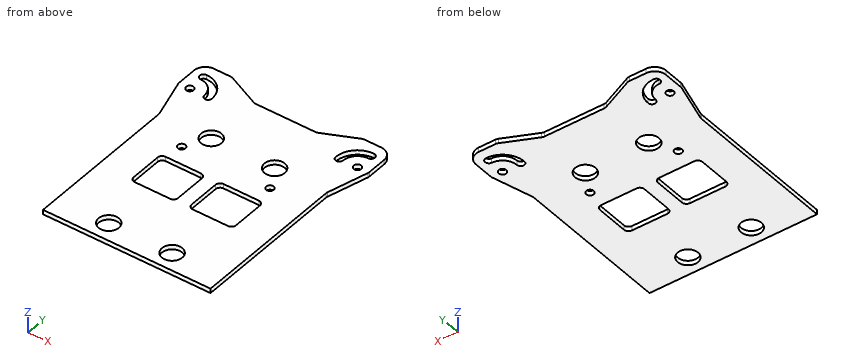
from build123d import *

# Parameters (mm, degrees)
F0_R     = 4.5
F0_R_2   = 1.65
F1_DEPTH = 2


with BuildPart() as f1:
    # F0 (on Top) → F1 (new body)
    with BuildSketch(Plane.XY):
        with BuildLine():
            Line((-29.655639, 60.219758), (-37, 60.219758))
            ThreePointArc((-37, 60.219758), (-40.535534, 58.755292), (-42, 55.219758))
            Line((-42, 55.219758), (-42, 46.628683))
            ThreePointArc((-42, 46.628683), (-41.972513, 46.223505), (-41.890554, 45.825751))
            Line((-41.890554, 45.825751), (-37.109446, 28.613764))
            ThreePointArc((-37.109446, 28.613764), (-37.027487, 28.216011), (-37, 27.810833))
            Line((-37, 27.810833), (-37, -39.780242))
            Line((-37, -39.780242), (37, -39.780242))
            Line((37, -39.780242), (37, 27.810833))
            ThreePointArc((37, 27.810833), (37.027487, 28.216011), (37.109446, 28.613764))
            Line((37.109446, 28.613764), (41.890554, 45.825751))
            ThreePointArc((41.890554, 45.825751), (41.972513, 46.223505), (42, 46.628683))
            Line((42, 46.628683), (42, 55.219758))
            ThreePointArc((42, 55.219758), (40.535534, 58.755292), (37, 60.219758))
            Line((37, 60.219758), (29.655639, 60.219758))
            ThreePointArc((29.655639, 60.219758), (29.015118, 60.150582), (28.404136, 59.946246))
            Line((28.404136, 59.946246), (14.345864, 53.493269))
            ThreePointArc((14.345864, 53.493269), (13.734882, 53.288933), (13.094361, 53.219758))
            Line((13.094361, 53.219758), (0, 53.219758))
            Line((0, 53.219758), (-13.094361, 53.219758))
            ThreePointArc((-13.094361, 53.219758), (-13.734882, 53.288933), (-14.345864, 53.493269))
            Line((-14.345864, 53.493269), (-28.404136, 59.946246))
            ThreePointArc((-28.404136, 59.946246), (-29.015118, 60.150582), (-29.655639, 60.219758))
        make_face()
        with Locations((-14, -31.780242)):
            Circle(F0_R, mode=Mode.SUBTRACT)
        with BuildLine():
            ThreePointArc((-5, 10.219758), (-3.585786, 9.633971), (-3, 8.219758))
            Line((-3, 8.219758), (-3, -5.780242))
            ThreePointArc((-3, -5.780242), (-3.585786, -7.194456), (-5, -7.780242))
            Line((-5, -7.780242), (-20.6, -7.780242))
            ThreePointArc((-20.6, -7.780242), (-22.014214, -7.194456), (-22.6, -5.780242))
            Line((-22.6, -5.780242), (-22.6, 8.219758))
            ThreePointArc((-22.6, 8.219758), (-22.014214, 9.633971), (-20.6, 10.219758))
            Line((-20.6, 10.219758), (-5, 10.219758))
        make_face(mode=Mode.SUBTRACT)
        with Locations((14, -31.780242)):
            Circle(F0_R, mode=Mode.SUBTRACT)
        with BuildLine():
            Line((3, -5.780242), (3, 8.219758))
            ThreePointArc((3, 8.219758), (3.585786, 9.633971), (5, 10.219758))
            Line((5, 10.219758), (20.6, 10.219758))
            ThreePointArc((20.6, 10.219758), (22.014214, 9.633971), (22.6, 8.219758))
            Line((22.6, 8.219758), (22.6, -5.780242))
            ThreePointArc((22.6, -5.780242), (22.014214, -7.194456), (20.6, -7.780242))
            Line((20.6, -7.780242), (5, -7.780242))
            ThreePointArc((5, -7.780242), (3.585786, -7.194456), (3, -5.780242))
        make_face(mode=Mode.SUBTRACT)
        with Locations((-19.5, 18.219758)):
            Circle(F0_R_2, mode=Mode.SUBTRACT)
        with Locations((-14, 28.219758)):
            Circle(F0_R, mode=Mode.SUBTRACT)
        with Locations((-37, 46.219758)):
            Circle(F0_R_2, mode=Mode.SUBTRACT)
        with BuildLine():
            ThreePointArc((-37, 55.869758), (-30.17642, 53.043338), (-27.35, 46.219758))
            ThreePointArc((-27.35, 46.219758), (-29, 44.569758), (-30.65, 46.219758))
            ThreePointArc((-30.65, 46.219758), (-32.509872, 50.709886), (-37, 52.569758))
            ThreePointArc((-37, 52.569758), (-38.65, 54.219758), (-37, 55.869758))
        make_face(mode=Mode.SUBTRACT)
        with Locations((19.5, 18.219758)):
            Circle(F0_R_2, mode=Mode.SUBTRACT)
        with Locations((14, 28.219758)):
            Circle(F0_R, mode=Mode.SUBTRACT)
        with Locations((37, 46.219758)):
            Circle(F0_R_2, mode=Mode.SUBTRACT)
        with BuildLine():
            ThreePointArc((30.65, 46.219758), (29, 44.569758), (27.35, 46.219758))
            ThreePointArc((27.35, 46.219758), (30.17642, 53.043338), (37, 55.869758))
            ThreePointArc((37, 55.869758), (38.65, 54.219758), (37, 52.569758))
            ThreePointArc((37, 52.569758), (32.509872, 50.709886), (30.65, 46.219758))
        make_face(mode=Mode.SUBTRACT)
    extrude(amount=F1_DEPTH)


solid = f1.part
Verification items for the finished model (mm, model axes). Coordinates: 2 decimals unless noted, no trailing zeros. Order: outer loops, then holes, each group sorted by start corner. A loop starts at its lowest first (then second) coordinate and runs counter-clockwise, first axis right, second up. Notation, with made-up numbers: M 36,29.25 L 50,29.25 A13 cw 50,54.25 Z; hole C 7.5,66 d5. An arc over 180 degrees is marked long. Write each question's results on one line, items separated by ' | '.
1) Scan lines: line 1 along X through (y, z) = (5.5, 0.8); line 2 along Y through (x, z) = (19.5, 1.25); line 3 along Y through (x, z) = (-7.5, 1.2). Record each from-to range of solid material in increasing order. Write a range as [from, to].
Solved:
line 1: x = [-37, -22.6], [-3, 3], [22.6, 37] | line 2: y = [-39.78, -7.78], [10.22, 16.57], [19.87, 55.86] | line 3: y = [-39.78, -7.78], [10.22, 53.22]
2) Section check A-A on y = 4. Record the cut outline in (x, z), plus the area to 3 significant figures.
Solved:
outline: M -37,0 L -22.6,0 L -22.6,2 L -37,2 Z; M -3,0 L 3,0 L 3,2 L -3,2 Z; M 22.6,0 L 37,0 L 37,2 L 22.6,2 Z | area: 69.6 mm²
3) Section check D-D on x = 32. Record the cut outline in (y, z), plus the area to 3 significant figures.
Solved:
outline: M -39.78,0 L 50.13,0 L 50.13,2 L -39.78,2 Z; M 54.47,0 L 60.22,0 L 60.22,2 L 54.47,2 Z | area: 191 mm²
4) Gauge pin test, flat ends, axial feed: pin 1 Ø14.5 at (x, y) = (14, 28.22) entering from -Z; pin 2 Ø1 at (y, z) = (-22, 1) entering from -X; pin 3 Ø1 at (y, z) = (-2, 1) entering from +X. Record the tip position at first contact, or that the pin passes through.
Solved:
pin 1: stops at z = 0 | pin 2: stops at x = -37 | pin 3: stops at x = 37
5) Section check C-C on y = 30. Record the cut outline in (x, z).
Solved:
outline: M -37.49,0 L -18.13,0 L -18.13,2 L -37.49,2 Z; M -9.87,0 L 9.87,0 L 9.87,2 L -9.87,2 Z; M 18.13,0 L 37.49,0 L 37.49,2 L 18.13,2 Z
6) Section check B-B on x = -8. Record the cut outline in (y, z), plus the area to 3 significant figures.
Solved:
outline: M -39.78,0 L -7.78,0 L -7.78,2 L -39.78,2 Z; M 10.22,0 L 53.22,0 L 53.22,2 L 10.22,2 Z | area: 150 mm²
